from build123d import *

# Parameters (mm, degrees)
SKETCH_1_W      = 50
SKETCH_1_H      = 8
EXTRUDE_2_DEPTH = 30
SKETCH_5_R      = 5
EXTRUDE_3_DEPTH = 5


with BuildPart() as part:
    # 扫描1: sweep along a path in 草图2
    with BuildLine(Plane(origin=(0, 0, 0), x_dir=(0, 0, -1), z_dir=(1, 0, 0))) as sweep_1_path:
        Line((0, 55.298323556), (-160, 55.298323556))
    # 草图1 → 扫描1 (sweep)
    with BuildSketch(Plane.XY):
        Rectangle(SKETCH_1_W, SKETCH_1_H)
    sweep(path=sweep_1_path.line)

    # 草图4 → 凸台-拉伸2 (add)
    with BuildSketch(Plane.XY.offset(160)):
        with BuildLine():
            Line((15, 19), (25, 4))
            Line((25, 4), (-25, 4))
            Line((-25, 4), (-15, 19))
            ThreePointArc((-15, 19), (0, 34), (15, 19))
        make_face()
    extrude(amount=-EXTRUDE_2_DEPTH)

    # 草图5 → 凸台-拉伸3 (add)
    with BuildSketch(Plane.XY.offset(160)):
        with Locations((0, 19)):
            Circle(SKETCH_5_R)
    extrude(amount=EXTRUDE_3_DEPTH)


solid = part.part
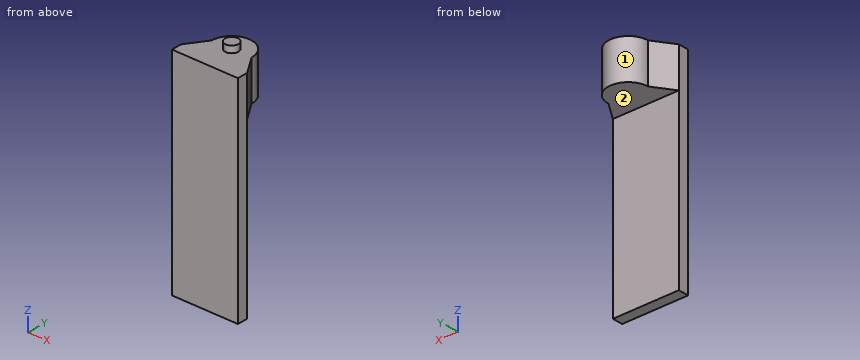
Can you work these out from the model? Positions are in its coordinate system, mm. Face numbers are marked on the shaded views. A direction names the side the tool comes from. Give positions to 0.01 mm unless a question says otherwise; leave off trailing zeros. Write each loop counter-clockwise with the first axis right and the second up, starting at its lowest first coordinate (ties: lowest second). Pieces come first, ordered by that corner, then holes. Notation, with made-up numbers: M 76,55 L 132,55 A12 ccw 132,69 Z; hole C 60,-32.5 d3. An arc over 180 degrees is marked long. Answer in a Markdown table with one row per item. Add a question column.
Item 1: Imagine slicing it at B-B, the plane z = 41. Write out the boundary of the cut face in (x, y), plus the area to 3 significant figures.
Item 2: On a 3-axis mill with a long thin cutter (end or side, diameter ignored), from which of +Z, -Z, +X, -X, +Y, -Y can I reach the whole of each face in a straight line? I mean the marked faces 1 and 2. Say none if no direction works.
Item 3: Imagine slicing it at C-C, the plane y = 11. Write out the boundary of the cut face in (x, z), plus the area to 3 significant figures.
Item 4: For pin 1 Ø10 at (x, y) = (-1, 30) entering from -Z; pin 2 Ø10 at (x, z) = (19.5, 79) entering from +Y, each with a flat end and sliding along its axis, tell me the tip position at first contact or that it passes through.
Item 5: Imagine slicing it at A-A, the plane x = 0. Write out the boundary of the cut face in (y, z).
Item 6: Imagine slicing it at D-D, the plane x = -8. Write out the boundary of the cut face in (y, z), plus the area to 3 significant figures.
Item 7: Please list where these lines run through material, in increasing order: L1, parallel to Z at x = 1, y = 9; L2, parallel to Z at x = -2, y = 23; L3, parallel to Y at x = -5, z = 127.
Evaluation:
| question | item | result |
|---|---|---|
| 1 | outline | M -25,-4 L 25,-4 L 25,4 L -25,4 Z |
| 1 | area | 400 mm² |
| 2 | face 1 | +Z, -Z, +Y |
| 2 | face 2 | -Z, +X, -X, +Y |
| 3 | outline | M -20.33,130 L 20.33,130 L 20.33,160 L -20.33,160 Z |
| 3 | area | 1,220 mm² |
| 4 | pin 1 | stops at z = 130 |
| 4 | pin 2 | stops at y = 4 |
| 5 | outline | M -4,0 L 4,0 L 4,130 L 34,130 L 34,160 L 24,160 L 24,165 L 14,165 L 14,160 L -4,160 Z |
| 6 | outline | M -4,0 L 4,0 L 4,130 L 31.69,130 L 31.69,160 L -4,160 Z |
| 6 | area | 2,110 mm² |
| 7 | L1 | z = 130 to 160 |
| 7 | L2 | z = 130 to 165 |
| 7 | L3 | y = -4 to 4 |
